Source: CAD feature listing. Evaluate the final solid. Frame: model axes, mm. A direction names the side the tool comes from. Round coordinates to 2 decimals unless told otherwise and drop trailing zeros. Write each loop counter-clockwise with the first axis right and the second up, starting at its lowest first coordinate (ties: lowest second). Pieces come first, ordered by that corner, then holes.
```python
from build123d import *

# Parameters (mm, degrees)
BOSS_EXTRUDE1_DEPTH = 51
SKETCH2_W           = 17.735009552
SKETCH2_H           = 9.543683463
BOSS_EXTRUDE2_DEPTH = 1.4
BOSS_EXTRUDE3_START = -51
SKETCH2_2_W         = 17.735009552
SKETCH2_2_H         = 9.543683463
BOSS_EXTRUDE3_DEPTH = 1.4


with BuildPart() as part:
    # Sketch1 → Boss-Extrude1 (new body)
    with BuildSketch(Plane(origin=(0, 0, 0), x_dir=(1, 0, 0), z_dir=(0, 1, 0))):
        with BuildLine():
            Line((-6.860118192, 1.392400227), (-8.867504776, 1.392400227))
            Line((-8.867504776, 1.392400227), (-8.867504776, -8.151283236))
            Line((-8.867504776, -8.151283236), (8.867504776, -8.151283236))
            Line((8.867504776, -8.151283236), (8.867504776, 1.392400227))
            Line((8.867504776, 1.392400227), (6.860118192, 1.392400227))
            ThreePointArc((6.860118192, 1.392400227), (0, -7), (-6.860118192, 1.392400227))
        make_face()
    extrude(amount=BOSS_EXTRUDE1_DEPTH)

    # Sketch2 → Boss-Extrude2 (add)
    with BuildSketch(Plane.XZ):
        with Locations((0, 3.379441505)):
            Rectangle(SKETCH2_W, SKETCH2_H)
    extrude(amount=BOSS_EXTRUDE2_DEPTH)

    # Sketch2<2> → Boss-Extrude3 (add)
    with BuildSketch(Plane.XZ.offset(BOSS_EXTRUDE3_START)):
        with Locations((0, 3.379441505)):
            Rectangle(SKETCH2_2_W, SKETCH2_2_H)
    extrude(amount=-BOSS_EXTRUDE3_DEPTH)


solid = part.part
```
Q1. Section query D-D, the plane x = -6. Output: boundary loops of the cut face in (y, z).
Q2. Section query B-B, the plane x = 0. Output: boundary loops of the cut face in (y, z).
Q3. Section query C-C, the plane y = 35. Output: boundary loops of the cut face in (x, z).
Q4. Pin query (flat end, axial travel): P1, Ø2, axis at x = -1.5, y = 41, coming from the -Z side; P2, Ø3, axis at x = -0.5, y = 32.5, coming from the -Z side. Return the tip coordinate at first contact, or that it passes through.
Q5. Mould query, pull axis X, two halves, no side actions, for faces 1 (the face through (-8.868, 25, 3)), 2 (the face through (0, 0, 2)), 3 (the face through (0, -1.4, 3)). Classes: pulls with the +X half, pulls with the -X half, needs draft (parallel to the pull), parting line crosses it, or undercut.
Q6. Line query: line 1 (Y direction, x = -4.5, z = 4.75); line 2 (X direction, y = 25, z = 0); line 3 (Z direction, x = 0, y = 40). Output: solid intervals per line, ascending.
Q7. Section query A-A, the plane z = 0. Output: boundary loops of the cut face in (x, y).
Q8. Set-up query: faces 4 (the face through (0, 25, 7)), 5 (the face through (0, 52.4, 3)). Return all of +Z, -Z, +X, -X, +Y, -Y with unobstructed straight access to the full face (end or side cutting, diameter ignored); none if empty.
Filled in:
1. outline: (-1.4, -1.39) - (0, -1.39) - (0, 3.61) - (51, 3.61) - (51, -1.39) - (52.4, -1.39) - (52.4, 8.15) - (-1.4, 8.15) - close
2. outline: (-1.4, -1.39) - (0, -1.39) - (0, 7) - (51, 7) - (51, -1.39) - (52.4, -1.39) - (52.4, 8.15) - (-1.4, 8.15) - close
3. outline: (-8.87, -1.39) - (-6.86, -1.39) arc R7 cw (long way) to (6.86, -1.39) - (8.87, -1.39) - (8.87, 8.15) - (-8.87, 8.15) - close
4. P1: stops at z = 6.54
4. P2: stops at z = 6.71
5. face 1: pulls with the -X half
5. face 2: undercut
5. face 3: needs draft
6. line 1: y = -1.4 to 0, 51 to 52.4
6. line 2: x = -8.87 to -7, 7 to 8.87
6. line 3: z = 7 to 8.15
7. outline: (-8.87, -1.4) - (8.87, -1.4) - (8.87, 52.4) - (-8.87, 52.4) - close; hole (-7, 0) - (7, 0) - (7, 51) - (-7, 51) - close
8. face 4: none
8. face 5: +Z, -Z, +X, -X, +Y
